```python
from build123d import *

# Parameters (mm, degrees)
F0_R     = 20
F1_DEPTH = 10
F2_W     = 100
F2_H     = 10
F3_DEPTH = 80
F4_R     = 20
F4_W     = 100
F4_H     = 10
F5_DEPTH = 10
F6_R     = 20
F7_DEPTH = 25


with BuildPart() as f1:
    # F0 (on Front) → F1 (new body)
    with BuildSketch(Plane.XZ):
        with BuildLine():
            Line((-10, 120), (-110, 120))
            Line((-110, 120), (-110, 20))
            Line((-110, 20), (6.721551, -101.556899))
            ThreePointArc((6.721551, -101.556899), (92.513193, -102.339443), (91.37931, -16.551724))
            Line((91.37931, -16.551724), (-10, 80))
            Line((-10, 80), (-10, 120))
        make_face()
        with Locations((50, -60)):
            Circle(F0_R, mode=Mode.SUBTRACT)
    extrude(amount=F1_DEPTH)

    # F2 (on face) → F3 (join)
    with BuildSketch(Plane.XZ.offset(10)):
        with Locations((-60, 115)):
            Rectangle(F2_W, F2_H)
    extrude(amount=F3_DEPTH)

    # F4 (on face) → F5 (join)
    with BuildSketch(Plane.XZ.offset(90)):
        with BuildLine():
            Line((-10, 110), (-110, 110))
            Line((-110, 110), (-110, 20))
            Line((-110, 20), (6.721551, -101.556899))
            ThreePointArc((6.721551, -101.556899), (92.513193, -102.339443), (91.37931, -16.551724))
            Line((91.37931, -16.551724), (-10, 80))
            Line((-10, 80), (-10, 110))
        make_face()
        with Locations((50, -60)):
            Circle(F4_R, mode=Mode.SUBTRACT)
        with Locations((-60, 115)):
            Rectangle(F4_W, F4_H)
    extrude(amount=F5_DEPTH)

    # F6 (on face) → F7 (cut)
    with BuildSketch(Plane.XY.offset(120)):
        with Locations((-60, -50)):
            Circle(F6_R)
    extrude(amount=-F7_DEPTH, mode=Mode.SUBTRACT)


solid = f1.part
```
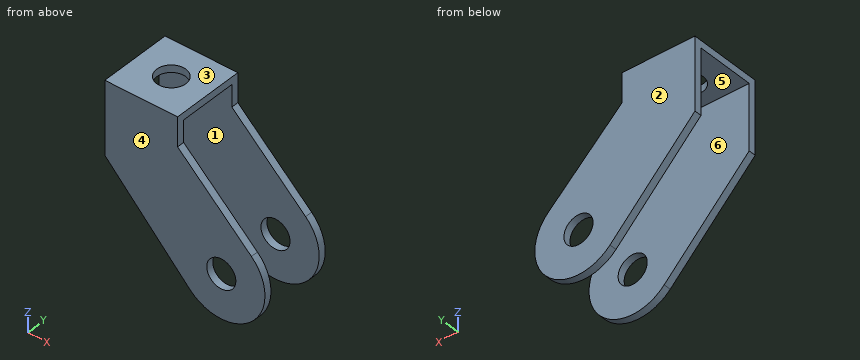
Geometry check sheet. Reference: the model listing, model coordinates, mm. Face numbers are marked on the shaded views. A direction names the side the tool comes from. Round coordinates to 2 decimals unless told otherwise and drop trailing zeros. Loops run counter-clockwise (first coordinate to the right, second up) from the corner with the lowest first, then second, coordinate; pieces in that order, holes last. Notation, with made-up numbers: (5.25, 83) -> (36.25, 83) arc R17 ccw to (36.25, 95) -> close; hole circle Ø3 at (-24, 18.5). An arc over 180 degrees is marked (long way). Use a Markdown table: item, result.
(1) Sectioned sample at C-C (y = -93). Enter the section's corners in (x, z).
Calculated:
| item | result |
|---|---|
| outline | (-110, 20) -> (6.72, -101.56) arc R60 ccw (long way) to (91.38, -16.55) -> (-10, 80) -> (-10, 120) -> (-110, 120) -> close; hole circle Ø40 at (50, -60) |
(2) Sectioned sample at A-A (z = 25). Enter the section's corners in (x, y), then the cut area to 4 significant figures.
Calculated:
| item | result |
|---|---|
| outline | (-110, -100) -> (47.75, -100) -> (47.75, -90) -> (-110, -90) -> close; (-110, -10) -> (47.75, -10) -> (47.75, 0) -> (-110, 0) -> close |
| area | 3,155 mm² |
(3) Sectioned sample at B-B (x = -60). Enter the section's corners in (y, z).
Calculated:
| item | result |
|---|---|
| outline | (-100, -32.07) -> (-90, -32.07) -> (-90, 110) -> (-70, 110) -> (-70, 120) -> (-100, 120) -> close; (-30, 110) -> (-10, 110) -> (-10, -32.07) -> (0, -32.07) -> (0, 120) -> (-30, 120) -> close |
(4) Go/stop test with a flat-tipped pin: P1, Ø4, axis at x = -27, y = -56, coming from the -Z side. Record where the tip stops, or that it passes through.
Calculated:
| item | result |
|---|---|
| P1 | z = 110 |
(5) Mould release check, pull along Y, two halves, no side actions. Record for the marked faces 3, 4, 5 and 6: released by +Y, released by -Y, zero draft, split by the parting line, or undercut.
Calculated:
| item | result |
|---|---|
| face 3 | zero draft |
| face 4 | released by -Y |
| face 5 | undercut |
| face 6 | undercut |
(6) Set-up check for the marked faces 1 and 2: record each of +Z, -Z, +X, -X, +Y, -Y from which the full face is reachable in a straight line by a thin tool's end or side.
Calculated:
| item | result |
|---|---|
| face 1 | -Z, +X, -X |
| face 2 | +Z, -Z, +X, -X, +Y |
(7) Scan lines: probe 1 along Y at (x, z) = (-60, 112.5); probe 2 along Y at (x, z) = (-100, 96); probe 3 along Z at (x, y) = (50, -3). Record each from-to range of solid material in increasing order.
Calculated:
| item | result |
|---|---|
| probe 1 | -100 to -70, -30 to 0 |
| probe 2 | -100 to -90, -10 to 0 |
| probe 3 | -120 to -80, -40 to 22.86 |
(8) Sectioned sample at D-D (x = 50). Enter the section's corners in (y, z).
Calculated:
| item | result |
|---|---|
| outline | (-100, -120) -> (-90, -120) -> (-90, -80) -> (-100, -80) -> close; (-100, -40) -> (-90, -40) -> (-90, 22.86) -> (-100, 22.86) -> close; (-10, -120) -> (0, -120) -> (0, -80) -> (-10, -80) -> close; (-10, -40) -> (0, -40) -> (0, 22.86) -> (-10, 22.86) -> close |
